Check sheet for the modelled part. Datum: model origin and axes. Units: mm. Give positions to 0.01 mm unless a question says otherwise; leave off trailing zeros. Order: outer loops, then holes, each group sorted by start corner. A loop starts at its lowest first (then second) coordinate and runs counter-clockwise, first axis right, second up.
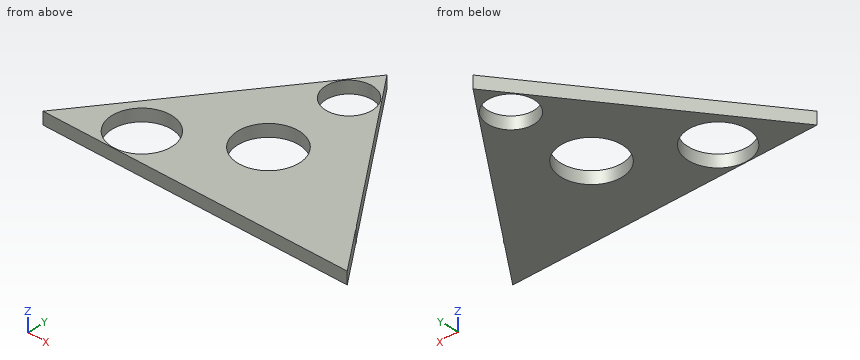
```python
from build123d import *

# Parameters (mm, degrees)
F0_R     = 14.5320210998
F0_R_2   = 11.3186574679
F1_DEPTH = 6


# Not quite as in the source:
# - the program builds the solid bodies; features that only make, move or delete a surface that nothing else refers to are left out


with BuildPart() as f1:
    # F0 (on Top) → F1 (new body)
    with BuildSketch(Plane.XY):
        with BuildLine():
            Line((0, 62.0833449066), (-46.019215806, 0))
            Line((-46.019215806, 0), (-74.3083804846, -38.1641872227))
            Line((-74.3083804846, -38.1641872227), (73.8562121987, -38.1641872227))
            Line((73.8562121987, -38.1641872227), (58.8761133365, -17.8311929182))
            ThreePointArc((58.8761133365, -17.8311929182), (60.0804416969, -20.9630848338), (60.4900211693, -24.2934599519))
            ThreePointArc((60.4900211693, -24.2934599519), (34.0337461373, -29.5218920802), (56.5122905135, -14.6226963362))
            Line((56.5122905135, -14.6226963362), (0, 62.0833449066))
        make_face()
        with Locations((-39.9468056858, -23.3477279544)):
            Circle(F0_R, mode=Mode.SUBTRACT)
        with BuildLine():
            ThreePointArc((14.9293226936, 0), (0, -14.9293226936), (-14.9293226936, 0))
            ThreePointArc((-14.9293226936, 0), (0, 14.9293226936), (14.9293226936, 0))
        make_face(mode=Mode.SUBTRACT)
        with Locations((0, 42.2229841352)):
            Circle(F0_R_2, mode=Mode.SUBTRACT)
        with BuildLine():
            ThreePointArc((58.8761133365, -17.8311929182), (57.8111056109, -16.140817186), (56.5122905135, -14.6226963362))
            Line((56.5122905135, -14.6226963362), (58.8761133365, -17.8311929182))
        make_face()
        with BuildLine():
            Line((58.8761133365, -17.8311929182), (56.5122905135, -14.6226963362))
            ThreePointArc((56.5122905135, -14.6226963362), (34.0337461373, -29.5218920802), (60.4900211693, -24.2934599519))
            ThreePointArc((60.4900211693, -24.2934599519), (60.0804416969, -20.9630848338), (58.8761133365, -17.8311929182))
        make_face()
    extrude(amount=F1_DEPTH)


solid = f1.part
```
(1) Cross-section at B-B on x = -46.5. Enter the section's corners in (y, z).
Response values:
outline: (-38.16, 0) - (-36.32, 0) - (-36.32, 6) - (-38.16, 6) - close; (-10.38, 0) - (-0.65, 0) - (-0.65, 6) - (-10.38, 6) - close
(2) Material ranges on L1, parallel to Y at x = 0, z = 4.7; L2, parallel to X at y = -4, z = 5.25; L3, parallel to X at y = -32, z = 2.4, recorded low to high.
Response values:
L1: y = -38.16 to -14.93, 14.93 to 30.9, 53.54 to 62.08
L2: x = -48.98 to -14.38, 14.38 to 48.69
L3: x = -69.74 to -51.62, -28.27 to 69.31
(3) Cross-section at D-D on x = 63. Enter the section's corners in (y, z).
Response values:
outline: (-38.16, 0) - (-23.43, 0) - (-23.43, 6) - (-38.16, 6) - close
(4) Gauge pin test, flat ends, axial feed: pin 1 Ø2 at (y, z) = (-22, 5) entering from -X; pin 2 Ø20.5 at (x, y) = (0, 42.22) entering from -Z. Record the tip position at first contact, or that the pin passes through.
Response values:
pin 1: stops at x = -63.07
pin 2: passes through
(5) Cross-section at A-A on y = 44.5. Enter the section's corners in (x, z), then the cut area to 3 significant figures.
Response values:
outline: (-13.03, 0) - (-11.09, 0) - (-11.09, 6) - (-13.03, 6) - close; (11.09, 0) - (12.95, 0) - (12.95, 6) - (11.09, 6) - close
area: 22.9 mm2
(6) Cross-section at C-C on z = 1.45. Enter the section's corners in (x, y).
Response values:
outline: (-74.31, -38.16) - (73.86, -38.16) - (58.88, -17.83) arc R13.74 ccw to (56.51, -14.62) - (0, 62.08) - close; hole circle Ø29.06 at (-39.95, -23.35); hole circle Ø29.86 at (0, 0); hole circle Ø22.64 at (0, 42.22)
